```python
from build123d import *

# Parameters (mm, degrees)
SKETCH1_R               = 44.45
BOSS_EXTRUDE1_DEPTH     = 12.7
SKETCH2_R               = 38.1
BOSS_EXTRUDE2_DEPTH     = 12.7
CUT_EXTRUDE1_DEPTH      = 68.7994469
CUT_EXTRUDE1_DEPTH_BACK = 68.7994469
SKETCH3_R               = 8.5725
CUT_EXTRUDE3_DEPTH      = 68.7994469
CUT_EXTRUDE3_DEPTH_BACK = 68.7994469
SKETCH4_R               = 17.78
SKETCH5_R               = 3.175
CUT_EXTRUDE4_DEPTH      = 12.7


with BuildPart() as part:
    # Sketch1 → Boss-Extrude1 (new body)
    with BuildSketch(Plane.XY):
        Circle(SKETCH1_R)
    extrude(amount=BOSS_EXTRUDE1_DEPTH)

    # Sketch2 → Boss-Extrude2 (add)
    with BuildSketch(Plane.XY.offset(12.7)):
        Circle(SKETCH2_R)
    extrude(amount=BOSS_EXTRUDE2_DEPTH)

    # Sketch3 → Cut-Extrude1 (cut, two sides: drawn at the far end of the back side and taken through both)
    with BuildSketch(Plane.XY.offset(25.4).offset(-CUT_EXTRUDE1_DEPTH_BACK)):
        with Locations((0, 21.59)):
            Circle(SKETCH3_R)
    extrude(amount=CUT_EXTRUDE1_DEPTH + CUT_EXTRUDE1_DEPTH_BACK, mode=Mode.SUBTRACT)

    # Sketch4 → Cut-Extrude3 (cut, two sides: drawn at the far end of the back side and taken through both)
    with BuildSketch(Plane.XY.offset(25.4).offset(-CUT_EXTRUDE3_DEPTH_BACK)):
        with Locations((0, -12.7)):
            Circle(SKETCH4_R)
    extrude(amount=CUT_EXTRUDE3_DEPTH + CUT_EXTRUDE3_DEPTH_BACK, mode=Mode.SUBTRACT)

    # Sketch5 → Cut-Extrude4 (cut)
    with BuildSketch(Plane(origin=(0, 0, 0), x_dir=(-1, 0, 0), z_dir=(0, 0, -1))):
        with Locations((27.94, -12.7)):
            Circle(SKETCH5_R)
        with Locations((-27.94, -12.7)):
            Circle(SKETCH5_R)
    extrude(amount=-CUT_EXTRUDE4_DEPTH, mode=Mode.SUBTRACT)


solid = part.part
```
Design review of the part built by this model. Coordinates are the model's own, in mm. A direction names the side the tool comes from. Coordinates: 2 decimals unless noted, no trailing zeros. Order: outer loops, then holes, each group sorted by start corner. A loop starts at its lowest first (then second) coordinate and runs counter-clockwise, first axis right, second up.
1) Take a section at A-A, the plane x = 0. Give the boundary of the cut face in (y, z).
2) Take a section at D-D, the plane z = 22.5. Give the boundary of the cut face in (x, y) (1 decimal), and give its area (3 significant figures).
3) Take a section at B-B, the plane y = -27. Give the boundary of the cut face in (x, z), and give its area (3 significant figures).
4) Clearance check with flat-ended pins moving along their axes: pin 1 (3 mm diameter, centred on x = 26.5, y = -12, fed in from -Z); pin 2 (8 mm diameter, centred on x = 20.5, z = 16, fed in from -Y); pin 3 (2 mm diameter, centred on y = -5.5, z = 15.5, fed in from +X). State where each tip first meets the part, or that it passes through.
5) Mouldability with a two-part tool opening along Y and no side actions: class faces 1 (the flat face through (33, 20, 12.7)), 2 (the cylindrical face through (42.397, 13.352, 6.261)), 3 (the cylindrical face through (-30.87, -13.92, 6.26)) as +Y half, -Y half, draft (parallel to the pull), parting line (faces both ways), or undercut.
6) Take a section at C-C, the plane z = 2.5. State how many separate pieces and enclosed holes the cut face has, and give its area (3 significant figures).
7) For faces 4 (the cylindrical face through (30.46, -14.63, 6.26)), 5 (the cylindrical face through (-30.235, -23.183, 18.961)), 6 (the cylindrical face through (-6.8, 16.37, 12.52)), list the 3-axis set-ups (+Z, -Z, +X, -X, +Y, -Y) from which the entire face can be reached by the end or side of a thin tool; tool diameter is ignored.
8) Wall thickness on line 1 along Y through (x, z) = (0, 9); line 2 along Y through (x, z) = (0, 13.5); line 3 along X through (y, z) = (21.59, 10.75): over which ranges is each line inside the solid? List them lowest first.
Returned:
1. outline: (-44.45, 0) - (-30.48, 0) - (-30.48, 25.4) - (-38.1, 25.4) - (-38.1, 12.7) - (-44.45, 12.7) - close; (5.08, 0) - (13.02, 0) - (13.02, 25.4) - (5.08, 25.4) - close; (30.16, 0) - (44.45, 0) - (44.45, 12.7) - (38.1, 12.7) - (38.1, 25.4) - (30.16, 25.4) - close
2. outline: circle Ø76.2 at (0, 0); hole circle Ø35.6 at (0, -12.7); hole circle Ø17.1 at (0, 21.6)
2. area: 3,340 mm2
3. outline: (-35.31, 0) - (-10.57, 0) - (-10.57, 25.4) - (-26.88, 25.4) - (-26.88, 12.7) - (-35.31, 12.7) - close; (10.57, 0) - (35.31, 0) - (35.31, 12.7) - (26.88, 12.7) - (26.88, 25.4) - (10.57, 25.4) - close
3. area: 1,040 mm2
4. pin 1: stops at z = 12.7
4. pin 2: stops at y = -40.54
4. pin 3: stops at x = 37.83
5. face 1: draft
5. face 2: parting line
5. face 3: undercut
6. separate pieces: 1
6. enclosed holes: 4
6. area: 4,920 mm2
7. face 4: -Z
7. face 5: +Z
7. face 6: +Z, -Z
8. line 1: y = -44.45 to -30.48, 5.08 to 13.02, 30.16 to 44.45
8. line 2: y = -38.1 to -30.48, 5.08 to 13.02, 30.16 to 38.1
8. line 3: x = -38.85 to -8.57, 8.57 to 38.85
